```python
from build123d import *

# Parameters (mm, degrees)
SKETCH1_W           = 100
SKETCH1_H           = 25.4
SKETCH1_W_2         = 25.4
SKETCH1_H_2         = 150
SKETCH1_W_3         = 42.3
BOSS_EXTRUDE1_DEPTH = 25.4
BOSS_EXTRUDE2_DEPTH = 40
CUT_EXTRUDE2_DEPTH  = 30
FILLET1_R           = 10


with BuildPart() as part:
    # Sketch1 → Boss-Extrude1 (new body)
    with BuildSketch(Plane.XY):
        with Locations((-62.7, 62.3)):
            Rectangle(SKETCH1_W, SKETCH1_H)
        Rectangle(SKETCH1_W_2, SKETCH1_H_2)
        with Locations((-33.85, -62.3)):
            Rectangle(SKETCH1_W_3, SKETCH1_H)
    extrude(amount=BOSS_EXTRUDE1_DEPTH)

    # Sketch2 → Boss-Extrude2 (add)
    with BuildSketch(Plane(origin=(0, 75, 0), x_dir=(1, 0, 0), z_dir=(0, 1, 0))):
        with BuildLine():
            ThreePointArc((-94.696699141, -7.396699141), (-105.303300859, -7.396699141), (-105.303300859, -18.003300859))
            Line((-105.303300859, -18.003300859), (-94.696699141, -7.396699141))
        make_face()
        with BuildLine():
            Line((-94.696699141, -7.396699141), (-105.303300859, -18.003300859))
            ThreePointArc((-105.303300859, -18.003300859), (-97.129874257, -19.629096494), (-92.5, -12.7))
            ThreePointArc((-92.5, -12.7), (-93.070903506, -9.829874257), (-94.696699141, -7.396699141))
        make_face()
    extrude(amount=BOSS_EXTRUDE2_DEPTH)

    # Sketch3 → Cut-Extrude2 (cut)
    with BuildSketch(Plane.ZY.offset(55)):
        with BuildLine():
            ThreePointArc((20.2, -62.3), (19.629096494, -59.429874257), (18.003300859, -56.996699141))
            Line((18.003300859, -56.996699141), (7.396699141, -67.603300859))
            ThreePointArc((7.396699141, -67.603300859), (15.570125743, -69.229096494), (20.2, -62.3))
        make_face()
        with BuildLine():
            Line((7.396699141, -67.603300859), (18.003300859, -56.996699141))
            ThreePointArc((18.003300859, -56.996699141), (7.396699141, -56.996699141), (7.396699141, -67.603300859))
        make_face()
    extrude(amount=-CUT_EXTRUDE2_DEPTH, mode=Mode.SUBTRACT)

    # Fillet1
    fillet1_edges = [part.edges().sort_by_distance(p)[0] for p in [
        (12.7, 75, 12.7),
        (12.7, -75, 12.7),
        (-12.7, -49.6, 12.7),
        (-12.7, 49.6, 12.7),
    ]]
    fillet(fillet1_edges, radius=FILLET1_R)


solid = part.part
```
The model under review builds one solid part; all positions refer to its coordinate system, in mm. A direction names the side the tool comes from. Round coordinates to 2 decimals unless told otherwise and drop trailing zeros. Loops run counter-clockwise (first coordinate to the right, second up) from the corner with the lowest first, then second, coordinate; pieces in that order, holes last. Notation, with made-up numbers: (32, 1) -> (48, 1) arc R21 cw to (48, 25) -> close; hole circle Ø10 at (-30, 25). An arc over 180 degrees is marked (long way). Answer as a JSON object with one key per item and string values. Group by question number.
1) We need section A-A on z = 23.5. Write out the cut boundary in (x, y), then the cut area to 3 significant figures.
2) We need section C-C on y = 73. Write out the cut boundary in (x, z).
3) For pin 1 Ø12 at (y, z) = (-62, 14.5) entering from -X; pin 2 Ø4 at (x, z) = (-44.5, 5.5) entering from +Y; pin 3 Ø7.5 at (y, z) = (-2, 16) entering from -X, all flat-tipped, find the tip position at first contact; note any pin that passes through.
4) We need section B-B on x = -100. Write out the cut boundary in (y, z), then the cut area to 3 significant figures.
5) For line 1 (Y direction, x = -45, z = 15.25); line 2 (Y direction, x = -44, z = 23); line 3 (X direction, y = 22.5, z = 2.5), list the stretches that pass through material, from the lowest coordinate up. Write a range as [from, to].
6) For faces 1 (the face through (-9, 18, 25.4)), 2 (the face through (-68, 49.6, 13)), 3 (the face through (-55, -68, 18)), list the 3-axis set-ups (+Z, -Z, +X, -X, +Y, -Y) from which the entire face can be reached by the end or side of a thin tool; tool diameter is ignored.
7) Mouldability with a two-part tool opening along Y and no side actions: class faces 4 (the face through (-25, -62, 13)), 5 (the face through (-9, 18, 0)), 6 (the face through (-100, 115, 13)), 7 (the face through (-12.7, -1, 13)) as released by +Y, released by -Y, zero draft, split by the parting line, or undercut.
8) We need section D-D on y = 36. Write out the cut boundary in (x, z).
Result set:
{
 "1": {"outline": "(-112.7, 49.6) -> (-22.7, 49.6) arc R10 cw to (-12.7, 39.6) -> (-12.7, -39.6) arc R10 cw to (-22.7, -49.6) -> (-55, -49.6) -> (-55, -75) -> (2.7, -75) arc R10 ccw to (12.7, -65) -> (12.7, 65) arc R10 ccw to (2.7, 75) -> (-112.7, 75) -> close", "area": "7,420 mm²"},
 "2": {"outline": "(-112.7, 0) -> (8.7, 0) -> (8.7, 25.4) -> (-112.7, 25.4) -> close"},
 "3": {"pin 1": "x = -55", "pin 2": "y = 75", "pin 3": "x = -12.7"},
 "4": {"outline": "(49.6, 0) -> (75, 0) -> (75, 5.2) -> (115, 5.2) -> (115, 20.2) -> (75, 20.2) -> (75, 25.4) -> (49.6, 25.4) -> close", "area": "1,250 mm²"},
 "5": {"line 1": "[-75, -69.35], [-55.25, -49.6], [49.6, 75]", "line 2": "[-75, -49.6], [49.6, 75]", "line 3": "[-12.7, 12.7]"},
 "6": {"face 1": "+Z, +X, -X, +Y, -Y", "face 2": "+Z, -Z, -X", "face 3": "+Z, -Z, -X, -Y"},
 "7": {"face 4": "undercut", "face 5": "zero draft", "face 6": "released by +Y", "face 7": "undercut"},
 "8": {"outline": "(-12.7, 0) -> (12.7, 0) -> (12.7, 25.4) -> (-12.7, 25.4) -> close"}
}
